Autodesk Inventor part; units mm, degrees
ref_plane "YZ Plane" through (0, 0, 0) normal (1, 0, 0) x (0, 1, 0)
ref_plane "XZ Plane" through (0, 0, 0) normal (0, 1, 0) x (-1, 0, 0)
ref_plane "XY Plane" through (0, 0, 0) normal (0, 0, 1) x (1, 0, 0)
sketch "Sketch1" plane through (0, 0, 0) normal (0, 0, 1) x (1, 0, 0)
  line L0 (0, 38.481) -> (0, -17.526)
  line L1 (-142.24, 0) -> (142.24, 0)
  line L2 (101.6, 30.48) -> (-101.6, 30.48)
  line L3 (-101.6, 30.48) -> (-101.6, -9.525)
  line L4 (-101.6, -9.525) -> (101.6, -9.525)
  line L5 (101.6, -9.525) -> (101.6, 30.48)
  line L6 (101.6, 30.48) -> (-101.6, -9.525) construction
  line L7 (-101.6, 30.48) -> (101.6, -9.525) construction
  point P0 (0, 0)
  point P1 (0, 10.4775)
  point P2 (-76.2, 0)
  point P3 (-25.4, 0)
  point P4 (25.4, 0)
  point P5 (76.2, 0)
  point P6 (-76.2, 19.05)
  point P7 (-25.4, 19.05)
  point P8 (25.4, 19.05)
  point P9 (76.2, 19.05)
  dimension "d0" = 9.525
  dimension "d1" = 30.48
  dimension "d2" = 203.2
  dimension "d3" = 50.8
  dimension "d4" = 25.4
  dimension "d5" = 25.4
  dimension "d6" = 50.8
  dimension "d11" = 19.05
extrude "Extrusion1" add sketch "Sketch1" against normal blind 4.4958
hole "Hole1" at (-76.2, 0, 0) at (-25.4, 0, 0) at (25.4, 0, 0) at (76.2, 0, 0) direction (0, 0, -1) diameter 4.4958 end through all countersink diameter 9.398 countersink angle 90
hole "Hole2" at (-76.2, 19.05, 0) at (-25.4, 19.05, 0) at (25.4, 19.05, 0) at (76.2, 19.05, 0) direction (0, 0, -1) diameter 3.1242 end through all
fillet "Fillet1" radius 3.175 4 edges at (-101.6, 30.48, -2.2479) (101.6, 30.48, -2.2479) (101.6, -9.525, -2.2479) (-101.6, -9.525, -2.2479)
Source: CAD feature listing. Evaluate the final solid. Frame: model axes, mm. Coordinates: 2 decimals unless noted, no trailing zeros. Loops run counter-clockwise (first coordinate to the right, second up) from the corner with the lowest first, then second, coordinate; pieces in that order, holes last. Notation, with made-up numbers: (32, 56.5) - (43, 56.5) arc R29 cw to (43, 81.5) - close; hole circle Ø10 at (6.25, -11.75). An arc over 180 degrees is marked (long way). Answer as CSV lines item,"result".
1. Mould query, pull axis Y, two halves, no side actions, for faces 1 (the conical face through (-26.861, 1.906, -2.298)), 2 (the flat face through (-1, 11, -4.496)), 3 (the flat face through (-1, -9.525, -2)). Classes: released by +Y, released by -Y, zero draft, split by the parting line, or undercut.
Established:
face 1,"undercut"
face 2,"zero draft"
face 3,"released by -Y"
2. Section B-B (z = -0.85). Count the separate pieces of the cut face and the enclosed holes in it, then the cut area to 3 significant figures.
Established:
separate pieces,"1"
enclosed holes,"8"
area,"7,900 mm2"
3. Contact query for a flat-ended pin moving along its axis: pin 1 (2.5 mm diameter, centred on x = -25.4, y = 0, fed in from +Z). Output: stop coordinate, or through.
Established:
pin 1,"passes through"
4. Section A-A (y = 0). Return loops of the section in (x, z).
Established:
outline,"(-101.6, -4.5) - (-78.45, -4.5) - (-78.45, -2.45) - (-80.9, 0) - (-101.6, 0) - close; (-73.95, -4.5) - (-27.65, -4.5) - (-27.65, -2.45) - (-30.1, 0) - (-71.5, 0) - (-73.95, -2.45) - close; (-23.15, -4.5) - (23.15, -4.5) - (23.15, -2.45) - (20.7, 0) - (-20.7, 0) - (-23.15, -2.45) - close; (27.65, -4.5) - (73.95, -4.5) - (73.95, -2.45) - (71.5, 0) - (30.1, 0) - (27.65, -2.45) - close; (78.45, -4.5) - (101.6, -4.5) - (101.6, 0) - (80.9, 0) - (78.45, -2.45) - close"
5. Ray query, line 1 (X direction, y = 19.05, z = -3.35); line 2 (Y direction, x = 25.4, z = -3.8) (3 decimals); line 3 (X direction, y = 18.5, z = -1.35). Return the intervals inside material, ascending.
Established:
line 1,"x = -101.6 to -77.76, -74.64 to -26.96, -23.84 to 23.84, 26.96 to 74.64, 77.76 to 101.6"
line 2,"y = -9.525 to -2.248, 2.248 to 17.488, 20.612 to 30.48"
line 3,"x = -101.6 to -77.66, -74.74 to -26.86, -23.94 to 23.94, 26.86 to 74.74, 77.66 to 101.6"
